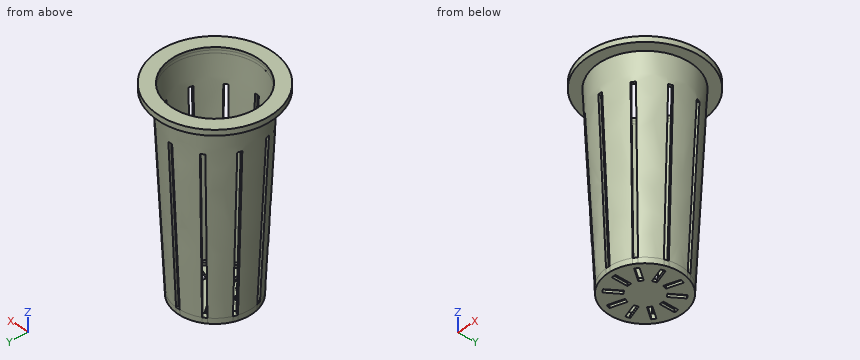
from build123d import *

# Parameters (mm, degrees)
F2_T     = -1.27
F3_DEPTH = 1.27
F5_R     = 20.32
F6_DEPTH = 25.4
F7_W     = 1.905
F7_H     = 19.812
F8_DEPTH = 76.2


with BuildPart() as f1:
    # F0 (on Front) → F1 (revolve)
    with BuildSketch(Plane.XZ):
        Polygon((0, 2.54), (0, 0), (14.732, 0), (17.272, 0), (17.3953714286, 2.54), align=None)
        Polygon((0, 88.9), (0, 2.54), (17.3953714286, 2.54), (21.59, 88.9), align=None)
        Polygon((0, 91.44), (0, 88.9), (21.59, 88.9), (26.67, 88.9), (26.67, 91.44), align=None)
    revolve(axis=Axis((0, 0, 44.45), (0, 0, 1)))

    # F2
    f2_openings = [f1.faces().sort_by_distance(p)[0] for p in [
        (0, 0, 91.44),
    ]]
    offset(amount=F2_T, openings=f2_openings, kind=Kind.INTERSECTION)

    # F3 (add): a face of the model
    f3_faces = [f1.faces().sort_by_distance(p)[0] for p in [
        (-24.6815795103, 0, 90.17),
    ]]
    extrude(f3_faces, amount=F3_DEPTH)

    # F5 (on offset) → F6 (cut)
    with BuildSketch(Plane.XY.offset(88.9)):
        Circle(F5_R)
    extrude(amount=F6_DEPTH, mode=Mode.SUBTRACT)

    # F7 (on Top) → F8 (cut)
    with BuildSketch(Plane.XY):
        Polygon((0.9525, -27.178), (0.9525, -7.366), (0, -7.366), (-0.9525, -7.366), (-0.9525, -27.178), align=None)
        Polygon((5.2068558942, -5.3647039539), (3.6656785199, -6.4844348595), (15.3108799383, -22.5126795521), (16.8520573126, -21.3929486464), align=None)
        Polygon((7.4723698113, -1.2449737892), (6.883692437, -3.0567364527), (25.7260241378, -9.1789811453), (26.3147015121, -7.3672184818), align=None)
        Polygon((6.883692437, 3.4195935956), (7.4723698113, 1.6078309321), (26.3147015121, 7.7300756246), (25.7260241378, 9.5418382882), align=None)
        Polygon((3.6656785199, 6.8472920024), (5.2068558942, 5.7275610967), (16.8520573126, 21.7558057893), (15.3108799383, 22.8755366949), align=None)
        with Locations((0, 17.6348571429)):
            Rectangle(F7_W, F7_H)
        Polygon((-5.2068558942, 5.7275610967), (-3.6656785199, 6.8472920024), (-15.3108799383, 22.8755366949), (-16.8520573126, 21.7558057893), align=None)
        Polygon((-7.4723698113, 1.6078309321), (-6.883692437, 3.4195935956), (-25.7260241378, 9.5418382882), (-26.3147015121, 7.7300756246), align=None)
        Polygon((-6.883692437, -3.0567364527), (-7.4723698113, -1.2449737892), (-26.3147015121, -7.3672184818), (-25.7260241378, -9.1789811453), align=None)
        Polygon((-3.6656785199, -6.4844348595), (-5.2068558942, -5.3647039539), (-16.8520573126, -21.3929486464), (-15.3108799383, -22.5126795521), align=None)
    extrude(amount=F8_DEPTH, mode=Mode.SUBTRACT)

    # F9 (on Front) → F10 (revolve)
    with BuildSketch(Plane.XZ):
        Polygon((14.8553677996, 2.54), (14.732, 0), (17.272, 0), (17.3953678, 2.54), align=None)
    revolve(axis=Axis((0, 0, 1.27), (0, 0, 1)))


solid = f1.part
Here's how the part is built. I have some questions about the finished solid (model axes, mm). Give positions to 0.01 mm unless a question says otherwise; leave off trailing zeros. Answer as a JSON object with one key per item and string values. Group by question number.
Item 1: Imagine slicing it at A-A on x = 0. Give the number of separate pieces and of enclosed holes in the cut face, then the cut area to 3 significant figures.
Item 2: I need wall thicknesses on L1, parallel to Y at x = 0, z = 90.55; L2, parallel to X at y = 11, z = 25; L3, parallel to Y at x = 0, z = 88. Which ranges of each line are inside material? Lowest first, please.
Item 3: Will these pins go through, and if not, where does the flat tip stop? pin 1 (8 mm diameter, centred on y = 19, z = 44.5, fed in from +X); pin 2 (1.4 mm diameter, centred on y = -11.5, z = 0.5, fed in from +X); pin 3 (1.1 mm diameter, centred on x = 12, y = -16.5, fed in from -Z).
Answer list:
{
 "1": {"separate pieces": "5", "enclosed holes": "0", "area": "96.4 mm2"},
 "2": {"L1": "y = -26.67 to -20.38, 20.38 to 26.67", "L2": "x = -14.86 to -13.24, 13.24 to 14.86", "L3": "y = -21.55 to -20.27, 20.27 to 21.55"},
 "3": {"pin 1": "stops at x = 12.37", "pin 2": "stops at x = 13.51", "pin 3": "stops at z = 76.2"}
}
